Input: part model. Units: mm. Frame: model coordinates. A direction names the side the tool comes from. Round coordinates to 2 decimals unless told otherwise and drop trailing zeros. Loops run counter-clockwise (first coordinate to the right, second up) from the corner with the lowest first, then second, coordinate; pieces in that order, holes last. Notation, with made-up numbers: (85.25, 40) -> (130.25, 40) arc R32 ccw to (130.25, 77) -> close; hole circle Ø1 at (21, -5). An arc over 180 degrees is marked (long way). Answer in a Markdown table with one row per item. Add a question column.
Q1. Section B-B, the plane x = 0. Output: boundary loops of the cut face in (y, z), and give its area (3 significant figures).
Q2. Section A-A, the plane z = -1.5. Output: boundary loops of the cut face in (x, y).
Q3. Mould query, pull axis X, two halves, no side actions, for faces 1 (the face through (-40, -16, -1)), 2 (the face through (11.503, 24.054, 4.028)), 3 (the face through (-29.9, -11.96, 5.1)). Classes: pulls with the +X half, pulls with the -X half, needs draft (parallel to the pull), parting line crosses it, or undercut.
Q4. Ray query, L1, parallel to X at y = 3.9, z = -2.5; L2, parallel to Y at x = 15, z = -3.5; L3, parallel to X at y = 23.9, z = 3.35. Return the intervals inside material, ascending. Write a range as from..to.
Q5. Section D-D, the plane x = 15. Output: boundary loops of the cut face in (y, z), and give its area (3 significant figures).
Q6. Section C-C, the plane y = -1.1. Output: boundary loops of the cut face in (x, z), and give its area (3 significant figures).
Q7. Pin query (flat end, axial travel): pin 1 (1 mm diameter, centred on x = -21, z = 3.5, fed in from +Y); pin 2 (2 mm diameter, centred on y = 9, z = -1.5, fed in from -X); pin 3 (6.5 mm diameter, centred on x = 15, y = 3.9, fed in from +Z); pin 4 (2.5 mm diameter, centred on x = 15, y = 23.9, fed in from -Z). Return the tip coordinate at first contact, or that it passes through.
Q8. Reachability of faces 4 (the face through (20, 14, -1)), 5 (the face through (11.503, 4.054, 4.028)), 6 (the face through (-20, 15, -1)) from +Z, -Z, +X, -X, +Y, -Y: full face, straight path, thin tool, end or side. Return the list, or none.
Autodesk Inventor part; units mm, degrees
ref_plane "YZ Plane" through (0, 0, 0) normal (1, 0, 0) x (0, 1, 0)
ref_plane "XZ Plane" through (0, 0, 0) normal (0, 1, 0) x (-1, 0, 0)
ref_plane "XY Plane" through (0, 0, 0) normal (0, 0, 1) x (1, 0, 0)
sketch "Sketch1" plane through (0, 0, 0) normal (0, 0, 1) x (1, 0, 0)
  line L0 (-40, -40) -> (40, -40)
  line L1 (40, -40) -> (40, 40)
  line L2 (40, 40) -> (-40, 40)
  line L3 (-40, 40) -> (-40, -40)
  line L4 (-40, -40) -> (40, 40) construction
  line L5 (40, -40) -> (-40, 40) construction
  point P0 (0, 0)
  dimension "d0" = 80
  dimension "d1" = 80
extrude "Extrusion1" add sketch "Sketch1" along normal blind 6
sketch "Sketch2" plane through (0, 0, 0) normal (0, 0, -1) x (-1, 0, 0)
  arc A0 (37, -21.1) -> (40, -18.1) centre (37, -18.1) ccw
  line L0 (37, -21.1) -> (-37, -21.1)
  arc A1 (-40, -18.1) -> (-37, -21.1) centre (-37, -18.1) ccw
  line L1 (-40, -14.1) -> (-40, -18.1)
  arc A2 (-37, -11.1) -> (-40, -14.1) centre (-37, -14.1) ccw
  line L2 (-23, -11.1) -> (-37, -11.1)
  arc A3 (-23, -11.1) -> (-20, -8.1) centre (-23, -8.1) ccw
  line L3 (-20, -8.1) -> (-20, 37)
  arc A4 (-17, 40) -> (-20, 37) centre (-17, 37) ccw
  line L4 (17, 40) -> (-17, 40)
  arc A5 (20, 37) -> (17, 40) centre (17, 37) ccw
  line L5 (20, 37) -> (20, -8.1)
  arc A6 (20, -8.1) -> (23, -11.1) centre (23, -8.1) ccw
  line L6 (37, -11.1) -> (23, -11.1)
  arc A7 (40, -14.1) -> (37, -11.1) centre (37, -14.1) ccw
  line L7 (40, -14.1) -> (40, -18.1)
  circle A8 centre (15, 3.9) radius 2
  circle A9 centre (-15, 3.9) radius 2
  circle A10 centre (15, 23.9) radius 2
  circle A11 centre (-15, 23.9) radius 2
  line L8 (12.1, 32) -> (12.1, -13.1)
  line L9 (-12.1, 32) -> (12.1, 32)
  line L10 (-12.1, -13.1) -> (-12.1, 32)
  line L11 (12.1, -13.1) -> (-12.1, -13.1)
  circle A12 centre (0, -1.1) radius 7.5
  line L12 (-40, -40) -> (40, -40)
  line L13 (40, -40) -> (40, 40)
  line L14 (40, 40) -> (-40, 40)
  line L15 (-40, 40) -> (-40, -40)
  line L16 (-40, -40) -> (40, 40) construction
  line L17 (40, -40) -> (-40, 40) construction
  line L18 (-40, 40) -> (40, 40)
  line L19 (40, 40) -> (40, -40)
  line L20 (-40, -40) -> (-40, 40)
  line L21 (40, -40) -> (-40, -40)
  point P0 (0, 0)
  point P1 (0, 0)
  point P2 (-40, -18.1)
extrude "Extrusion2" cut sketch "Sketch2" against normal blind 6 contours A0 L13 L12 L15 A1 L0 | A7 L6 A6 L5 A5 L14 L13 | L15 L14 A4 L3 A3 L2 A2 | A8 | A9 | A10 | A11 | A12
sketch "Sketch3" plane through (0, 0, 0) normal (0, 0, -1) x (-1, 0, 0)
  arc A0 (37, -21.1) -> (40, -18.1) centre (37, -18.1) ccw
  line L0 (37, -21.1) -> (-37, -21.1)
  arc A1 (-40, -18.1) -> (-37, -21.1) centre (-37, -18.1) ccw
  line L1 (-40, -14.1) -> (-40, -18.1)
  arc A2 (-37, -11.1) -> (-40, -14.1) centre (-37, -14.1) ccw
  line L2 (-23, -11.1) -> (-37, -11.1)
  arc A3 (-23, -11.1) -> (-20, -8.1) centre (-23, -8.1) ccw
  line L3 (-20, -8.1) -> (-20, 37)
  arc A4 (-17, 40) -> (-20, 37) centre (-17, 37) ccw
  line L4 (17, 40) -> (-17, 40)
  arc A5 (20, 37) -> (17, 40) centre (17, 37) ccw
  line L5 (20, 37) -> (20, -8.1)
  arc A6 (20, -8.1) -> (23, -11.1) centre (23, -8.1) ccw
  line L6 (37, -11.1) -> (23, -11.1)
  arc A7 (40, -14.1) -> (37, -11.1) centre (37, -14.1) ccw
  line L7 (40, -14.1) -> (40, -18.1)
  circle A8 centre (15, 3.9) radius 2
  circle A9 centre (-15, 3.9) radius 2
  circle A10 centre (15, 23.9) radius 2
  circle A11 centre (-15, 23.9) radius 2
  line L8 (12.1, 32) -> (12.1, -13.1)
  line L9 (-12.1, 32) -> (12.1, 32)
  line L10 (-12.1, -13.1) -> (-12.1, 32)
  line L11 (12.1, -13.1) -> (-12.1, -13.1)
  point P0 (0, 0)
extrude "Extrusion3" add sketch "Sketch3" along normal blind 5
sketch "Sketch4" plane through (0, 0, 6) normal (0, 0, 1) x (1, 0, 0)
  circle A0 centre (0, -1.1) radius 7.5
  circle A1 centre (0, -1.1) radius 11
  point P0 (0, 0)
  dimension "d8" = 22
extrude "Extrusion4" cut sketch "Sketch4" against normal through all
fillet "Fillet1" radius 3 16 edges at (-19.1213, 39.1213, 6) (-20, 14.45, 6) (-20.8787, -10.2213, 6) (-30, -11.1, 6) (-39.1213, -11.9787, 6) (-40, -16.1, 6) (-39.1213, -20.2213, 6) (0, -21.1, 6) (39.1213, -20.2213, 6) (40, -16.1, 6) (39.1213, -11.9787, 6) (30, -11.1, 6) (20.8787, -10.2213, 6) (20, 14.45, 6) (19.1213, 39.1213, 6) (0, 40, 6)
sketch "Sketch5" plane through (0, 0, 6) normal (0, 0, 1) x (1, 0, 0)
  circle A0 centre (-15, 23.9) radius 2
  line L0 (-17, 3.9) -> (-17, 23.9)
  circle A1 centre (-15, 3.9) radius 2
  line L1 (-17, -8.1) -> (-17, 3.9)
  arc A2 (-23, -14.1) -> (-17, -8.1) centre (-23, -8.1) ccw
  line L2 (-37, -14.1) -> (-23, -14.1)
  line L3 (-37, -18.1) -> (-37, -14.1)
  line L4 (37, -18.1) -> (-37, -18.1)
  line L5 (37, -14.1) -> (37, -18.1)
  line L6 (23, -14.1) -> (37, -14.1)
  arc A3 (17, -8.1) -> (23, -14.1) centre (23, -8.1) ccw
  line L7 (17, 3.9) -> (17, -8.1)
  circle A4 centre (15, 3.9) radius 2
  line L8 (17, 23.9) -> (17, 3.9)
  circle A5 centre (15, 23.9) radius 2
  line L9 (17, 37) -> (17, 23.9)
  line L10 (-17, 37) -> (17, 37)
  line L11 (-17, 23.9) -> (-17, 37)
  circle A6 centre (0, -1.1) radius 11
  circle A7 centre (-15, 23.9) radius 3.5
  circle A8 centre (15, 23.9) radius 3.5
  circle A9 centre (-15, 3.9) radius 3.5
  circle A10 centre (15, 3.9) radius 3.5
  point P0 (0, 0)
  dimension "d12" = 7
  dimension "d13" = 7
  dimension "d14" = 7
  dimension "d15" = 7
extrude "Extrusion5" cut sketch "Sketch5" against normal blind 4 contours L11 A7 L0 | L0 A7 L11 | A9 L1 L0 | L0 L1 A9 | A8 L8 L9 | L9 L8 A8 | A10 L7 L8 | L8 L7 A10
properties part number "stopper_motor_bracket_cover"
Answer block:
| question | item | result |
|---|---|---|
| 1 | outline | (-21.1, -5) -> (-13.1, -5) -> (-13.1, 0) -> (-12.1, 0) -> (-12.1, 6) -> (-18.1, 6) arc R3 ccw to (-21.1, 3) -> close; (9.9, 0) -> (32, 0) -> (32, -5) -> (40, -5) -> (40, 3) arc R3 ccw to (37, 6) -> (9.9, 6) -> close |
| 1 | area | 311 mm^2 |
| 2 | outline | (-40, -18.1) arc R3 ccw to (-37, -21.1) -> (37, -21.1) arc R3 ccw to (40, -18.1) -> (40, -14.1) arc R3 ccw to (37, -11.1) -> (23, -11.1) arc R3 cw to (20, -8.1) -> (20, 37) arc R3 ccw to (17, 40) -> (-17, 40) arc R3 ccw to (-20, 37) -> (-20, -8.1) arc R3 cw to (-23, -11.1) -> (-37, -11.1) arc R3 ccw to (-40, -14.1) -> close; hole circle Ø4 at (-15, 3.9); hole circle Ø4 at (-15, 23.9); hole (-12.1, -13.1) -> (12.1, -13.1) -> (12.1, 32) -> (-12.1, 32) -> close; hole circle Ø4 at (15, 3.9); hole circle Ø4 at (15, 23.9) |
| 3 | face 1 | pulls with the -X half |
| 3 | face 2 | undercut |
| 3 | face 3 | needs draft |
| 4 | L1 | -20..-17, -13..-12.1, 12.1..13, 17..20 |
| 4 | L2 | -21.1..1.9, 5.9..21.9, 25.9..40 |
| 4 | L3 | -19.98..-18.5, -11.5..11.5, 18.5..19.98 |
| 5 | outline | (-21.1, -5) -> (1.9, -5) -> (1.9, 2) -> (0.4, 2) -> (0.4, 6) -> (-18.1, 6) arc R3 ccw to (-21.1, 3) -> close; (5.9, -5) -> (21.9, -5) -> (21.9, 2) -> (20.4, 2) -> (20.4, 6) -> (7.4, 6) -> (7.4, 2) -> (5.9, 2) -> close; (25.9, -5) -> (40, -5) -> (40, 3) arc R3 ccw to (37, 6) -> (27.4, 6) -> (27.4, 2) -> (25.9, 2) -> close |
| 5 | area | 556 mm^2 |
| 6 | outline | (-20, -5) -> (-12.1, -5) -> (-12.1, 0) -> (-11, 0) -> (-11, 6) -> (-17, 6) arc R3 ccw to (-20, 3) -> close; (11, 0) -> (12.1, 0) -> (12.1, -5) -> (20, -5) -> (20, 3) arc R3 ccw to (17, 6) -> (11, 6) -> close |
| 6 | area | 183 mm^2 |
| 7 | pin 1 | y = -9.82 |
| 7 | pin 2 | x = -20 |
| 7 | pin 3 | z = 2 |
| 7 | pin 4 | through |
| 8 | face 4 | +Z, -Z, +X, +Y |
| 8 | face 5 | +Z |
| 8 | face 6 | +Z, -Z, -X, +Y |
